Model file for the job. Use its own axes, mm. A direction names the side the tool comes from. Give positions to 0.01 mm unless a question says otherwise; leave off trailing zeros. Loops run counter-clockwise (first coordinate to the right, second up) from the corner with the lowest first, then second, coordinate; pieces in that order, holes last. Notation, with made-up numbers: M 77,4 L 131,4 A25 ccw 131,41 Z; hole C 85,4 d4. An arc over 180 degrees is marked long. Use CSV: the item, a comma, the result in double quotes. Start each with the question number.
(1) Flat gauge pins, fed straight in: P1, Ø3, axis at x = -3, z = 48, coming from the +Y side; P2, Ø4, axis at x = 10.5, z = 38, coming from the +Y side; P3, Ø3, axis at x = 0, z = 40, coming from the -Y side. Where does each tip first touch, or does it go through?
(2) Slice it at D-D on z = 6. List the corners of the cut face in (x, y).
(3) Tool access for faces 1 (the face through (-2.539, -19.334, 52.479)), 2 (the face through (-10.316, -7.91, 35.882)): list every direction of +Z, -Z, +X, -X, +Y, -Y with a clear straight run to the whole face (end or side of a thin tool).
(4) Slice it at A-A on x = 0. List the corners of the cut face in (y, z).
(5) Wall check: line 1 along Y through (x, z) = (0, 32); line 2 along Z through (x, y) = (3, -15); line 3 along X through (y, z) = (5, 19). Give the ranges that are in metal, low to high. Write a range as from..to.
(6) Slice it at C-C on z = 39. List the corners of the cut face in (x, y).
(7) Two-plate mould, pull along Y, no slides. Class faces 3 (the face through (0, 0, 17.25)), 4 (the face through (6.691, 12.864, 25.143)), 5 (the face through (0, 15, 51)): pulls with the +Y half, pulls with the -Y half, needs draft (parallel to the pull), parting line crosses it, or undercut.
Autodesk Inventor part; units mm, degrees
ref_plane "YZ Plane" through (0, 0, 0) normal (1, 0, 0) x (0, 1, 0)
ref_plane "XZ Plane" through (0, 0, 0) normal (0, 1, 0) x (-1, 0, 0)
ref_plane "XY Plane" through (0, 0, 0) normal (0, 0, 1) x (1, 0, 0)
sketch "Sketch1" plane through (0, 0, 0) normal (0, 0, 1) x (1, 0, 0)
  circle A0 centre (0, 0) radius 14.5
  dimension "d0" = 29
extrude "Extrusion1" add sketch "Sketch1" along normal blind 51
sketch "Sketch2" plane through (0, 0, 51) normal (0, 0, 1) x (1, 0, 0)
  circle A0 centre (0, 0) radius 19.5
  circle A1 centre (0, 0) radius 14.5
  dimension "d3" = 5
extrude "Extrusion2" add sketch "Sketch2" along normal blind 3 contours A0 | A1
sketch "Sketch4" plane through (0, 0, 54) normal (0, 0, 1) x (1, 0, 0)
  circle A0 centre (0, 0) radius 13
  dimension "d44" = 26
extrude "Extrusion3" cut sketch "Sketch4" against normal blind 36.75
equation "\"d0\" = r_usboutlet"
equation "\"wl_panel\" = 285"
equation "\"t_panel\" = 8"
equation "\"r_button\" = 8"
equation "\"l_stereo\" = 178"
equation "\"d_stereo\" = 177"
equation "\"w_label\" = 15"
equation "\"r_labelscrew\" = 2.5"
equation "\"ro_labelscrew\" = 5"
equation "\"l_buttontobutton\" = 25"
equation "\"r_usboutlet\" = 29"
equation "\"l_fastener_button\" = 19"
properties part number "usb_outlet" material "Thermoplastic Resin"
Reply:
1,P1,"stops at y = 14.42"
1,P2,"stops at y = 11.75"
1,P3,"stops at y = -14.5"
2,outline,"C 0,0 d29"
3,face 1,"+Z, -Z"
3,face 2,"+Z"
4,outline,"M -19.5,51 L -14.5,51 L -14.5,0 L 14.5,0 L 14.5,51 L 19.5,51 L 19.5,54 L 13,54 L 13,17.25 L -13,17.25 L -13,54 L -19.5,54 Z"
5,line 1,"y = -14.5..-13, 13..14.5"
5,line 2,"z = 51..54"
5,line 3,"x = -13.61..-12, 12..13.61"
6,outline,"C 0,0 d29; hole C 0,0 d26"
7,face 3,"undercut"
7,face 4,"parting line crosses it"
7,face 5,"needs draft"
